from build123d import *

# Parameters (mm, degrees)
BOSS_EXTRUDE2_DEPTH = 50
CUT_EXTRUDE1_DEPTH  = 42.2
CIRPATTERN1_COUNT   = 3


with BuildPart() as part:
    # Sketch3 → Boss-Extrude2 (new body)
    with BuildSketch(Plane(origin=(0, 0, 0), x_dir=(1, 0, 0), z_dir=(0, 1, 0))):
        Polygon((-21.1, -12.18209068), (-21.1, -175), (21.1, -175), (21.1, -12.18209068), (0, 0), align=None)
    boss_extrude2 = extrude(amount=BOSS_EXTRUDE2_DEPTH)

    # Sketch4 → Cut-Extrude1 (cut)
    with BuildSketch(Plane.ZY.offset(21.1)):
        Polygon((175, 0), (104.277828473, 50), (175, 50), align=None)
    cut_extrude1 = extrude(amount=-CUT_EXTRUDE1_DEPTH, mode=Mode.SUBTRACT)

    # CirPattern1: Boss-Extrude2, Cut-Extrude1 ×3 about axis
    cirpattern1_axis = Axis((0, 0, 0), (0, 1, 0))
    for i in range(1, CIRPATTERN1_COUNT):
        add(boss_extrude2.rotate(cirpattern1_axis, i * 360 / CIRPATTERN1_COUNT))
        add(cut_extrude1.rotate(cirpattern1_axis, i * 360 / CIRPATTERN1_COUNT), mode=Mode.SUBTRACT)


solid = part.part
Input: part model. Units: mm. Frame: model coordinates. A direction names the side the tool comes from. Coordinates: 2 decimals unless noted, no trailing zeros. Order: outer loops, then holes, each group sorted by start corner. A loop starts at its lowest first (then second) coordinate and runs counter-clockwise, first axis right, second up. Notation, with made-up numbers: M 47.25,2.5 L 76.25,2.5 A9 ccw 76.25,13.5 Z; hole C -7,-14 d2. An arc over 180 degrees is marked long. Write item = value, one per line. Start each with the question number.
(1) First-contact query: P1, Ø4, axis at x = -1, y = 10, coming from the +Z side; P2, Ø10, axis at y = 11, z = 23.5, coming from the +X side; P3, Ø4, axis at y = 30.5, z = 98, coming from the -X side. Flat tips, straight axial feed; report the tip coordinate or a pass-through.
(2) Section B-B on z = 92. Output: boundary loops of the cut face in (x, y).
(3) Section C-C on x = 132.5. Output: boundary loops of the cut face in (y, z).
(4) Reachability of faces 1 (the flat face through (-21.1, 25, 74)), 2 (the flat face through (4, 50, 1)), 3 (the flat face through (-53.848, 24.65, -55.453)) from +Z, -Z, +X, -X, +Y, -Y: full face, straight path, thin tool, end or side. Return the list, or none.
(5) Pull-direction query (X, two-part tool) for faces 4 (the flat face through (21.1, 25, 77)), 5 (the flat face through (55.82, 24.65, -56.59)), 6 (the flat face through (-121.21, 24.65, -70.32)); classes: released by +X, released by -X, zero draft, split by the parting line, or undercut.
(6) Section D-D on x = 97. Output: boundary loops of the cut face in (y, z).
(7) Section A-A on y = 37. Output: boundary loops of the cut face in (x, z).
(8) Line query: line 1 along X through (y, z) = (4.5, 70.5); line 2 along X through (y, z) = (28.5, -62); line 3 along X through (y, z) = (31.5, -71). Output: solid intervals per line, ascending. Write a range as [from, to].
Result set:
q1.P1 = 163.68
q1.P2 = 21.1
q1.P3 = -21.1
q2.outline = M -21.1,0 L 21.1,0 L 21.1,50 L -21.1,50 Z
q3.outline = M 0,-100.86 L 6.94,-100.86 L 24.17,-52.13 L 0,-52.13 Z
q4.face_1 = +Z, -X, +Y, -Y
q4.face_2 = +Z, -Z, +X, -X, +Y
q4.face_3 = -Z, +Y, -Y
q5.face_4 = released by +X
q5.face_5 = undercut
q5.face_6 = released by -X
q6.outline = M 0,-80.37 L 35.92,-80.37 L 50,-40.55 L 50,-31.64 L 0,-31.64 Z
q7.outline = M -116.78,-43.06 L -95.68,-79.61 L 0,-24.36 L 95.68,-79.61 L 116.78,-43.06 L 21.1,12.18 L 21.1,122.67 L -21.1,122.67 L -21.1,12.18 Z
q8.line_1 = [-21.1, 21.1]
q8.line_2 = [-119.73, -65.19], [65.19, 119.73]
q8.line_3 = [-109.63, -80.78], [80.78, 109.63]
